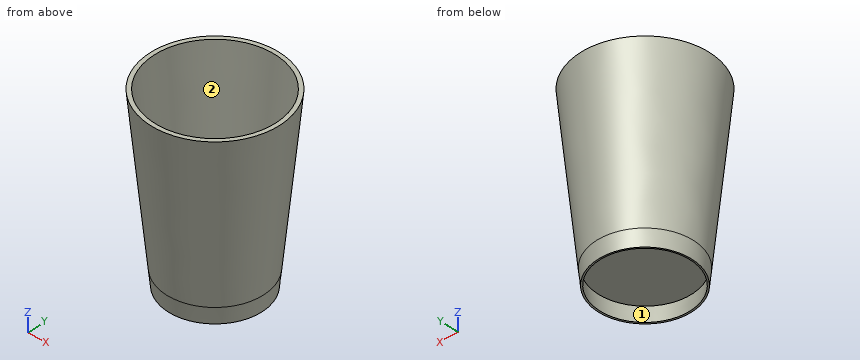
from build123d import *

# Parameters (mm, degrees)
F2_T = -2.5


with BuildPart() as f1:
    # F0 (on Front) → F1 (revolve)
    with BuildSketch(Plane.XZ):
        Polygon((40, 100), (0, 100), (0, 0), (28.995012, 0), (30, 0), align=None)
        Polygon((29.004963, -9.950372), (30, 0), (28.995012, 0), (28.009926, -9.850868), align=None)
    revolve(axis=Axis((0, 0, 50), (0, 0, -1)))

    # F2
    f2_openings = [f1.faces().sort_by_distance(p)[0] for p in [
        (0, 0, 100),
    ]]
    offset(amount=F2_T, openings=f2_openings)


solid = f1.part
For this review, take the finished solid that the model builds, in its own axes (mm). Face numbers are marked on the shaded views. Round coordinates to 2 decimals unless told otherwise and drop trailing zeros. Loops run counter-clockwise (first coordinate to the right, second up) from the corner with the lowest first, then second, coordinate; pieces in that order, holes last. Notation, with made-up numbers: (83.25, 88) - (134.25, 88) arc R19 ccw to (134.25, 119) - close; hole circle Ø3 at (45.5, 34). An arc over 180 degrees is marked (long way). One line per item, written item: value. Start each with the question number.
Item 1: The part is to be moulded in two halves that separate along X. For the marked faces 1 and 2, say which applies: +X half, -X half, draft (parallel to the pull), parting line (faces both ways), or undercut.
Item 2: For L1, parallel to Z at x = 5.5, y = -21; L2, parallel to X at y = 31.5, z = 90.5; L3, parallel to Y at x = -24, z = 20, list the stretches that pass through material, from the lowest coordinate up.
Item 3: Take a section at B-B (z = 70). Give the boundary of the cut face in (x, y), plus the area to 3 significant figures.
Item 4: Take a section at A-A (z = 48). Give the boundary of the cut face in (x, y), plus the area to 3 significant figures.
Item 5: Clearance check with flat-ended pins moving along their axes: pin 1 Ø1.5 at (x, z) = (-16, 65) entering from +Y; pin 2 Ø1.5 at (y, z) = (8.5, 35.5) entering from -X; pin 3 Ø3 at (y, z) = (23, 63) entering from +X. State where each tip first meets the part, or that it passes through.
Answer below:
1. face 1: undercut
1. face 2: undercut
2. L1: z = 0 to 2.5
2. L2: x = -23.08 to -18.51, 18.51 to 23.08
2. L3: y = -21.17 to -17.13, 17.13 to 21.17
3. outline: circle Ø74 at (0, 0); hole circle Ø68.98 at (0, 0)
3. area: 564 mm2
4. outline: circle Ø69.6 at (0, 0); hole circle Ø64.58 at (0, 0)
4. area: 530 mm2
5. pin 1: stops at y = 33.17
5. pin 2: stops at x = -32.66
5. pin 3: stops at x = 29.26
